from build123d import *

# Parameters (mm, degrees)
SKETCH_1_W          = 44
SKETCH_1_H          = 25.4
EXTRUDE_1_DEPTH     = 77.5
CUT_EXTRUDE_1_DEPTH = 82.556973951
SKETCH_3_R          = 2.5
CUT_EXTRUDE_2_DEPTH = 6
CUT_EXTRUDE_3_DEPTH = 15
SKETCH_5_R          = 2.5
CUT_EXTRUDE_4_DEPTH = 1
CHAMFER_1_SIZE      = 1


with BuildPart() as part:
    # 草图1 → 凸台-拉伸1 (new body)
    with BuildSketch(Plane(origin=(0, 0, 0), x_dir=(1, 0, 0), z_dir=(0, 1, 0))):
        Rectangle(SKETCH_1_W, SKETCH_1_H)
    extrude(amount=EXTRUDE_1_DEPTH)

    # 草图2 → 切除-拉伸1 (cut, through all)
    with BuildSketch(Plane.XZ):
        Polygon((8, -1.2), (-8, -1.2), (-10, -3.2), (-10, -7.7), (-7, -10.7), (-7, -12.7), (7, -12.7), (7, -10.7), (10, -7.7), (10, -3.2), align=None)
    extrude(amount=-CUT_EXTRUDE_1_DEPTH, mode=Mode.SUBTRACT)

    # 草图3 → 切除-拉伸2 (cut)
    with BuildSketch(Plane.XY.offset(12.7)):
        with Locations((-16, 20.75)):
            Circle(SKETCH_3_R)
        with Locations((-16, 56.75)):
            Circle(SKETCH_3_R)
        with Locations(Location((16, 56.75, 0), (0, 0, 180))):
            Circle(SKETCH_3_R)
        with Locations(Location((16, 20.75, 0), (0, 0, 180))):
            Circle(SKETCH_3_R)
    extrude(amount=-CUT_EXTRUDE_2_DEPTH, mode=Mode.SUBTRACT)

    # 草图4 → 切除-拉伸3 (cut)
    with BuildSketch(Plane(origin=(0, 77.5, 0), x_dir=(1, 0, 0), z_dir=(0, 1, 0))):
        Polygon((22, -12.7), (22, 12.7), (7, 12.7), (7, 10.7), (10, 7.7), (10, 3.2), (8, 1.2), (-8, 1.2), (-10, 3.2), (-10, 7.7), (-7, 10.7), (-7, 12.7), (-22, 12.7), (-22, -12.7), align=None)
        Polygon((21.9, -12.6), (21.9, 12.6), (7.1, 12.6), (7.1, 10.741421356), (10.1, 7.741421356), (10.1, 3.158578644), (8.041421356, 1.1), (-8.041421356, 1.1), (-10.1, 3.158578644), (-10.1, 7.741421356), (-7.1, 10.741421356), (-7.1, 12.6), (-21.9, 12.6), (-21.9, -12.6), align=None, mode=Mode.SUBTRACT)
    cut_extrude_3 = extrude(amount=-CUT_EXTRUDE_3_DEPTH, mode=Mode.SUBTRACT)

    # 镜向1: 切除-拉伸3 across plane
    add(cut_extrude_3.mirror(Plane.ZX.offset(38.75)), mode=Mode.SUBTRACT)

    # 草图5 → 切除-拉伸4 (cut)
    with BuildSketch(Plane.XY.offset(12.6)):
        with Locations((0, 7.5)):
            Circle(SKETCH_5_R)
        with Locations(Location((0, 70, 0), (0, 0, 180))):
            Circle(SKETCH_5_R)
    extrude(amount=-CUT_EXTRUDE_4_DEPTH, mode=Mode.SUBTRACT)

    # 倒角1
    chamfer_1_edges = [part.edges().sort_by_distance(p)[0] for p in [
        (21.9, 0, 0),
        (14.5, 0, -12.6),
        (7.1, 0, -11.670710678),
        (8.6, 0, -9.241421356),
        (10.1, 0, -5.45),
        (9.070710678, 0, -2.129289322),
        (0, 0, -1.1),
        (-9.070710678, 0, -2.129289322),
        (-10.1, 0, -5.45),
        (-8.6, 0, -9.241421356),
        (-7.1, 0, -11.670710678),
        (-14.5, 0, -12.6),
        (-21.9, 0, 0),
        (0, 0, 12.6),
        (21.9, 77.5, 0),
        (14.5, 77.5, -12.6),
        (7.1, 77.5, -11.670710678),
        (8.6, 77.5, -9.241421356),
        (10.1, 77.5, -5.45),
        (9.070710678, 77.5, -2.129289322),
        (0, 77.5, -1.1),
        (-9.070710678, 77.5, -2.129289322),
        (-10.1, 77.5, -5.45),
        (-8.6, 77.5, -9.241421356),
        (-7.1, 77.5, -11.670710678),
        (-14.5, 77.5, -12.6),
        (-21.9, 77.5, 0),
        (0, 77.5, 12.6),
    ]]
    chamfer(chamfer_1_edges, length=CHAMFER_1_SIZE)


solid = part.part
Model file for the job. Use its own axes, mm. A direction names the side the tool comes from. Round coordinates to 2 decimals unless told otherwise and drop trailing zeros. Loops run counter-clockwise (first coordinate to the right, second up) from the corner with the lowest first, then second, coordinate; pieces in that order, holes last. Notation, with made-up numbers: (41.25, 15) -> (96.25, 15) arc R20 ccw to (96.25, 54) -> close; hole circle Ø4 at (70, 81.5). An arc over 180 degrees is marked (long way). Answer as CSV lines item,"result". Start each with the question number.
1) Slice it at C-C (y = 56.75). List the corners of the cut face in (x, z), plus the area to 3 significant figures.
2) Slice it at A-A (y = 6). List the corners of the cut face in (x, z).
3) Mould opens along X. For faces 6 (the face through (-21.9, 8, 0)), 7 (the face through (-16, 57, 6.7)), 8 (the face through (21.9, 8, 0)) say: +X half, -X half, draft (parallel to the pull), parting line (faces both ways), or undercut.
4) Tool access for faces 1 (the face through (-14, 8, -12.6)), 2 (the face through (8.58, 7.9, -9.26)), 3 (the face through (-10.1, 70, -5)), 4 (the face through (16, 21, 6.7)), 5 (the face through (8.5, 38.4, -9.2)): list every direction of +Z, -Z, +X, -X, +Y, -Y with a clear straight run to the whole face (end or side of a thin tool).
5) Pin check, flat tips, straight feed: P1, Ø6.5, axis at x = 16, y = 56.75, coming from the +Z side; P2, Ø5.5, axis at x = 0.5, y = 7, coming from the +Z side; P3, Ø11, axis at x = -13.5, y = 6, coming from the -Z side; P4, Ø4.5, axis at x = 16, y = 20.75, coming from the +Z side. Stop position of each tip, or through.
6) Probe line 1 along Y through (x, z) = (0, 12.35); line 2 along X through (y, z) = (49.5, -11); line 3 along X through (y, z) = (51.5, -4.75). List the from-to ranges inside material, lowest first.
7) Slice it at B-B (x = 0). List the corners of the cut face in (y, z), plus the area to 3 significant figures.
8) Slice it at D-D (x = 16). List the corners of the cut face in (y, z), plus the area to 3 significant figures.
Filled in:
1,outline,"(-22, -12.7) -> (-7, -12.7) -> (-7, -10.7) -> (-10, -7.7) -> (-10, -3.2) -> (-8, -1.2) -> (8, -1.2) -> (10, -3.2) -> (10, -7.7) -> (7, -10.7) -> (7, -12.7) -> (22, -12.7) -> (22, 12.7) -> (18.5, 12.7) -> (18.5, 6.7) -> (13.5, 6.7) -> (13.5, 12.7) -> (-13.5, 12.7) -> (-13.5, 6.7) -> (-18.5, 6.7) -> (-18.5, 12.7) -> (-22, 12.7) -> close"
1,area,"853 mm2"
2,outline,"(-21.9, -12.6) -> (-7.1, -12.6) -> (-7.1, -10.74) -> (-10.1, -7.74) -> (-10.1, -3.16) -> (-8.04, -1.1) -> (8.04, -1.1) -> (10.1, -3.16) -> (10.1, -7.74) -> (7.1, -10.74) -> (7.1, -12.6) -> (21.9, -12.6) -> (21.9, 12.6) -> (2, 12.6) -> (2, 11.6) -> (-2, 11.6) -> (-2, 12.6) -> (-21.9, 12.6) -> close"
3,face 6,"-X half"
3,face 7,"undercut"
3,face 8,"+X half"
4,face 1,"-Z, +X, -X, -Y"
4,face 2,"-Y"
4,face 3,"+Y"
4,face 4,"+Z"
4,face 5,"+Y, -Y"
5,P1,"stops at z = 12.7"
5,P2,"stops at z = 12.6"
5,P3,"stops at z = -12.6"
5,P4,"stops at z = 6.7"
6,line 1,"y = 0.75 to 5, 10 to 67.5, 72.5 to 76.75"
6,line 2,"x = -22 to -7, 7 to 22"
6,line 3,"x = -22 to -10, 10 to 22"
7,outline,"(0, -0.1) -> (1, -1.1) -> (15, -1.1) -> (15, -1.2) -> (62.5, -1.2) -> (62.5, -1.1) -> (76.5, -1.1) -> (77.5, -0.1) -> (77.5, 11.6) -> (76.5, 12.6) -> (72.5, 12.6) -> (72.5, 11.6) -> (67.5, 11.6) -> (67.5, 12.6) -> (62.5, 12.6) -> (62.5, 12.7) -> (15, 12.7) -> (15, 12.6) -> (10, 12.6) -> (10, 11.6) -> (5, 11.6) -> (5, 12.6) -> (1, 12.6) -> (0, 11.6) -> close"
7,area,"1,060 mm2"
8,outline,"(0, -11.6) -> (1, -12.6) -> (15, -12.6) -> (15, -12.7) -> (62.5, -12.7) -> (62.5, -12.6) -> (76.5, -12.6) -> (77.5, -11.6) -> (77.5, 11.6) -> (76.5, 12.6) -> (62.5, 12.6) -> (62.5, 12.7) -> (59.25, 12.7) -> (59.25, 6.7) -> (54.25, 6.7) -> (54.25, 12.7) -> (23.25, 12.7) -> (23.25, 6.7) -> (18.25, 6.7) -> (18.25, 12.7) -> (15, 12.7) -> (15, 12.6) -> (1, 12.6) -> (0, 11.6) -> close"
8,area,"1,900 mm2"
